Build history of the part. All positions in model axes, mm. A direction names the side the tool comes from. Give positions to 0.01 mm unless a question says otherwise; leave off trailing zeros. Order: outer loops, then holes, each group sorted by start corner. A loop starts at its lowest first (then second) coordinate and runs counter-clockwise, first axis right, second up. Notation, with made-up numbers: (86, 82.25) -> (127, 82.25) arc R12 ccw to (127, 103.25) -> close; hole circle Ø8 at (50, 52.25). An arc over 180 degrees is marked (long way). One line per item, written item: value. Start each with the question number.
(1) Probe line 1 (X direction, y = 66.5, z = 2.2); line 2 (Y direction, x = 31.5, z = 1.6); line 3 (Y direction, x = 40.7, z = 1.95). List the from-to ranges inside material, lowest first.
(2) Saw through at B-B on y = 16. Give the cut face in (x, z), plus the area to 3 significant figures.
(3) Which spindle directions (+Z, -Z, +X, -X, +Y, -Y) get a long thin tool onto all of the face, cutting with end or side? Do faces 4 (the flat face through (42.25, 15, 1)), 5 (the flat face through (49, 10, 1)), 6 (the flat face through (23, 80, 1)). Say none if no direction does.
(4) Saw through at C-C on x = 9. Give the cut face in (y, z), plus the area to 3 significant figures.
(5) Pin check, flat tip, straight feed: pin 1 (1.5 mm diameter, centred on x = 0.5, z = 1.5, fed in from -Y). Stop position of the tip, or through.
(6) Saw through at D-D on y = 47.5. Give the cut face in (x, z).
(7) Two-plate mould, pull along X, no slides. Class faces 1 (the flat face through (-10, 45, 1)), 2 (the cylindrical face through (-4.65, 13.07, 1.48)), 3 (the flat face through (56, 45, 1)): +X half, -X half, draft (parallel to the pull), parting line (faces both ways), or undercut.
(8) Saw through at A-A on x = -4. Give the cut face in (y, z), plus the area to 3 significant figures.
```python
from build123d import *

# Parameters (mm, degrees)
F0_R     = 3
F0_R_2   = 2.5
F0_W     = 38.5
F0_H     = 20
F0_W_2   = 23
F0_H_2   = 29
F0_R_3   = 2.9306388833
F0_W_3   = 22.8
F1_DEPTH = 3


# Not quite as in the source:
# - a feature names something its author has since deleted; it is built from what else it names


with BuildPart() as f1:
    # F0 (on Top) → F1 (new body)
    with BuildSketch(Plane.XY):
        with BuildLine():
            ThreePointArc((-0.0987510204, 4.899238456), (1.4005055782, 1.429019202), (4.9002335876, 0))
            Line((4.9002335876, 0), (41.2, 0))
            ThreePointArc((41.2, 0), (44.7355339059, 1.4644660941), (46.2, 5))
            Line((46.2, 5), (46.2, 10))
            Line((46.2, 10), (51, 10))
            ThreePointArc((51, 10), (54.5355339059, 11.4644660941), (56, 15))
            Line((56, 15), (56, 30))
            Line((56, 30), (56, 75))
            ThreePointArc((56, 75), (54.5355339059, 78.5355339059), (51, 80))
            Line((51, 80), (-5, 80))
            ThreePointArc((-5, 80), (-8.5355339059, 78.5355339059), (-10, 75))
            Line((-10, 75), (-10, 30))
            Line((-10, 30), (-10, 15))
            ThreePointArc((-10, 15), (-8.5355339059, 11.4644660941), (-5, 10))
            Line((-5, 10), (-0.2015640213, 10))
            Line((-0.2015640213, 10), (-0.0987510204, 4.899238456))
        make_face()
        with Locations((-4, 16)):
            Circle(F0_R, mode=Mode.SUBTRACT)
        with Locations((5.5, 34.8868072033)):
            Circle(F0_R_2, mode=Mode.SUBTRACT)
        with Locations((23, 15)):
            Rectangle(F0_W, F0_H, mode=Mode.SUBTRACT)
        with Locations((50, 16)):
            Circle(F0_R, mode=Mode.SUBTRACT)
        with Locations((40.7, 34.8868072033)):
            Circle(F0_R_2, mode=Mode.SUBTRACT)
        with Locations((5.5, 54.5)):
            Rectangle(F0_W_2, F0_H_2, mode=Mode.SUBTRACT)
        with Locations((-4, 74)):
            Circle(F0_R_3, mode=Mode.SUBTRACT)
        with Locations((40.6, 54.5)):
            Rectangle(F0_W_3, F0_H_2, mode=Mode.SUBTRACT)
        with Locations((50, 74)):
            Circle(F0_R_3, mode=Mode.SUBTRACT)
    extrude(amount=F1_DEPTH)


solid = f1.part
```
Results below:
1. line 1: x = -10 to -6, 17 to 29.2, 52 to 56
1. line 2: y = 0 to 5, 25 to 40, 69 to 80
1. line 3: y = 0 to 5, 25 to 32.39, 37.39 to 40, 69 to 80
2. outline: (-10, 0) -> (-7, 0) -> (-7, 3) -> (-10, 3) -> close; (-1, 0) -> (3.75, 0) -> (3.75, 3) -> (-1, 3) -> close; (42.25, 0) -> (47, 0) -> (47, 3) -> (42.25, 3) -> close; (53, 0) -> (56, 0) -> (56, 3) -> (53, 3) -> close
2. area: 46.5 mm²
3. face 4: +Z, -Z
3. face 5: +Z, -Z, +X, -Y
3. face 6: +Z, -Z, +X, -X, +Y
4. outline: (0, 0) -> (5, 0) -> (5, 3) -> (0, 3) -> close; (25, 0) -> (40, 0) -> (40, 3) -> (25, 3) -> close; (69, 0) -> (80, 0) -> (80, 3) -> (69, 3) -> close
4. area: 93.0 mm²
5. pin 1: stops at y = 1.58
6. outline: (-10, 0) -> (-6, 0) -> (-6, 3) -> (-10, 3) -> close; (17, 0) -> (29.2, 0) -> (29.2, 3) -> (17, 3) -> close; (52, 0) -> (56, 0) -> (56, 3) -> (52, 3) -> close
7. face 1: -X half
7. face 2: undercut
7. face 3: +X half
8. outline: (10, 0) -> (13, 0) -> (13, 3) -> (10, 3) -> close; (19, 0) -> (40, 0) -> (40, 3) -> (19, 3) -> close; (69, 0) -> (71.07, 0) -> (71.07, 3) -> (69, 3) -> close; (76.93, 0) -> (80, 0) -> (80, 3) -> (76.93, 3) -> close
8. area: 87.4 mm²
